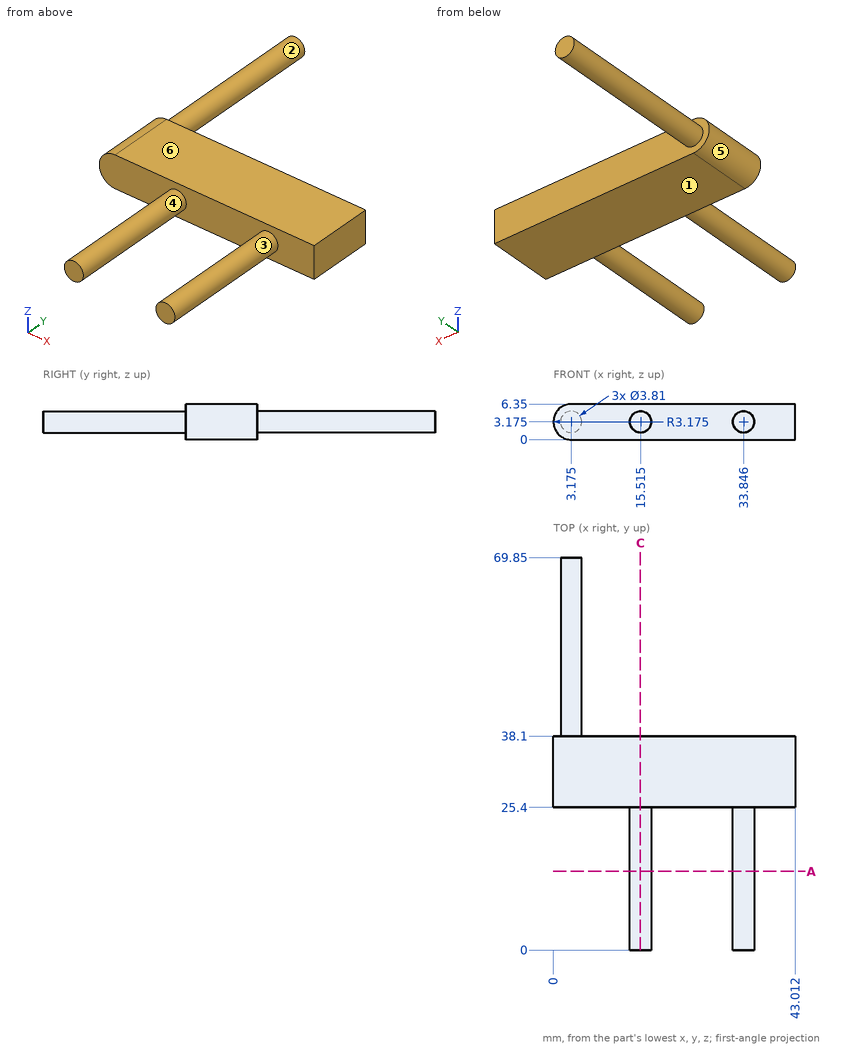
The figure shows three views and two pictorial views of one solid part (mm, origin at its lowest corner). Answer the questions. A direction names the side the tool comes from. Round coordinates to 2 decimals unless told otherwise and drop trailing zeros. Loops run counter-clockwise (first coordinate to the right, second up) from the corner with the lowest first, then second, coordinate; pieces in that order, holes last. Notation, with made-up numbers: (-12, -11) - (-7, -11) arc R9 cw to (-7, 3) - close; hole circle Ø11 at (66, 36.25). An arc over 180 degrees is marked (long way). One line per question, with ' | ' between items. Start each with the question number.
Q1. Flat-ended cylindrical pins translate along their axes: pin 1 (1 mm diameter, centred on y = 56, z = 2, fed in from +X); pin 2 (3 mm diameter, centred on x = 12, z = 2.5, fed in from -Y); pin 3 (4 mm diameter, centred on x = 32.5, y = 10, fed in from +Z). Find the tip coordinate at first contact, or state that the pin passes through.
Q2. For the marked faces 1 and 2, determine the directions among +Z, -Z, +X, -X, +Y, -Y from which every point of the face is accessible in a straight line to the end or side of a thin tool.
Q3. Section C-C on x = 15.5 is taken. Give the vertices of the cut face in (y, z), plus the area to 3 significant figures.
Q4. For a pull along X with two mould halves and no side action, classify the marked faces 3, 4, 5 and 6 as +X half, -X half, draft (parallel to the pull), parting line (faces both ways), or undercut.
Q5. Section A-A on y = 14 is taken. Give the vertices of the cut face in (x, z) (1 decimal), plus the area to 3 significant figures.
Q6. Find the intervals of material crossed by L1, parallel to Y at x = 16.5, z = 1; L2, parallel to Y at x = 4, z = 4; L3, parallel to Z at x = 3, y = 41, in increasing order.
Established:
1) pin 1: x = 4.96 | pin 2: y = 25.4 | pin 3: z = 5.08
2) face 1: -Z, +X, -X, +Y, -Y | face 2: +Y
3) outline: (0, 1.27) - (25.4, 1.27) - (25.4, 0) - (38.1, 0) - (38.1, 6.35) - (25.4, 6.35) - (25.4, 5.08) - (0, 5.08) - close | area: 177 mm²
4) face 3: undercut | face 4: undercut | face 5: -X half | face 6: draft
5) outline: circle Ø3.8 at (15.5, 3.2); circle Ø3.8 at (33.8, 3.2) | area: 22.8 mm²
6) L1: 25.4 to 38.1 | L2: 25.4 to 69.85 | L3: 1.28 to 5.07
